from build123d import *

# Parameters (mm, degrees)
SKETCH_2_R      = 2
EXTRUDE_1_DEPTH = 10


with BuildPart() as part:
    # Эскиз2 → Бобышка-Вытянуть1 (new body)
    with BuildSketch(Plane.XY):
        with BuildLine():
            Line((6.5, 0), (6.5, -14))
            Line((6.5, -14), (12.5, -14))
            Line((12.5, -14), (12.5, 18))
            Line((12.5, 18), (-17.5, 18))
            Line((-17.5, 18), (-17.5, -14))
            Line((-17.5, -14), (0.5, -14))
            Line((0.5, -14), (0.5, -6.480740698))
            ThreePointArc((0.5, -6.480740698), (-4.769696007, 4.415880433), (6.5, 0))
        make_face()
        with Locations((-11.5, 12)):
            Circle(SKETCH_2_R, mode=Mode.SUBTRACT)
        with Locations((-11.5, -9)):
            Circle(SKETCH_2_R, mode=Mode.SUBTRACT)
    extrude(amount=EXTRUDE_1_DEPTH)


solid = part.part
CAD build for the part. Positions are in the model's coordinates, mm. A direction names the side the tool comes from. Round coordinates to 2 decimals unless told otherwise and drop trailing zeros. Loops run counter-clockwise (first coordinate to the right, second up) from the corner with the lowest first, then second, coordinate; pieces in that order, holes last. Notation, with made-up numbers: (47.5, 26) - (106.5, 26) arc R33 cw to (106.5, 55) - close; hole circle Ø10 at (81.25, 57.25). An arc over 180 degrees is marked (long way). Put each result on its own line as item: value.
1. Slice it at B-B on x = -11.5. List the corners of the cut face in (y, z).
Geometry check:
outline: (-14, 0) - (-11, 0) - (-11, 10) - (-14, 10) - close; (-7, 0) - (10, 0) - (10, 10) - (-7, 10) - close; (14, 0) - (18, 0) - (18, 10) - (14, 10) - close
2. Slice it at C-C on z = 8. List the corners of the cut face in (x, y).
Geometry check:
outline: (-17.5, -14) - (0.5, -14) - (0.5, -6.48) arc R6.5 cw (long way) to (6.5, 0) - (6.5, -14) - (12.5, -14) - (12.5, 18) - (-17.5, 18) - close; hole circle Ø4 at (-11.5, -9); hole circle Ø4 at (-11.5, 12)
3. Two-plate mould, pull along X, no slides. Class faces 3 (the flat face through (-2, 18, 5)), 4 (the flat face through (12.5, 2, 5)), 5 (the cylindrical face through (-12.974, 13.352, 4.93)): released by +X, released by -X, zero draft, split by the parting line, or undercut.
Geometry check:
face 3: zero draft
face 4: released by +X
face 5: undercut
4. Slice it at D-D on x = 0. List the corners of the cut face in (y, z), and give its area (3 significant figures).
Geometry check:
outline: (-14, 0) - (-6.5, 0) - (-6.5, 10) - (-14, 10) - close; (6.5, 0) - (18, 0) - (18, 10) - (6.5, 10) - close
area: 190 mm²
5. 3-axis set-ups, long thin cutter, end or side, ignore diameter. For faces 1 (the flat face through (0.5, -10, 5)), 2 (the cylindrical face through (-12.974, -7.648, 4.93)): which of +Z, -Z, +X, -X, +Y, -Y reach the whole face in a straight line?
Geometry check:
face 1: +Z, -Z, -Y
face 2: +Z, -Z
6. Pin check, flat tip, straight feed: P1, Ø10.5, axis at x = 0, y = 0, coming from the -Z side. Stop position of the tip, or through.
Geometry check:
P1: through
7. Slice it at A-A on y = 12. List the corners of the cut face in (x, z).
Geometry check:
outline: (-17.5, 0) - (-13.5, 0) - (-13.5, 10) - (-17.5, 10) - close; (-9.5, 0) - (12.5, 0) - (12.5, 10) - (-9.5, 10) - close
8. Wall check: line 1 (Y direction, x = -11.5, z = 4); line 2 (Y direction, x = -10, z = 7.25); line 3 (Y direction, x = 0, z = 2.75). Give the ranges that are in metal, low to high.
Geometry check:
line 1: -14 to -11, -7 to 10, 14 to 18
line 2: -14 to -10.32, -7.68 to 10.68, 13.32 to 18
line 3: -14 to -6.5, 6.5 to 18
